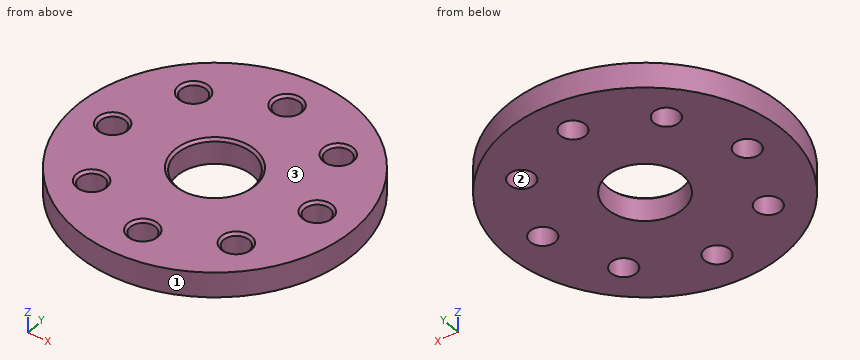
```python
from build123d import *

# Parameters (mm, degrees)
SKETCH1_R           = 11
BOSS_EXTRUDE1_DEPTH = 2
SKETCH3_R           = 3
CUT_EXTRUDE1_DEPTH  = 16.684387141
SKETCH4_R           = 1
CUT_EXTRUDE2_DEPTH  = 16.684387141
CHAMFER1_SIZE       = 0.2
CHAMFER2_SIZE       = 0.2
CIRPATTERN1_COUNT   = 8
CHAMFER4_SIZE       = 0.2
CHAMFER5_SIZE       = 0.2
CHAMFER6_SIZE       = 0.2


with BuildPart() as part:
    # Sketch1 → Boss-Extrude1 (new body)
    with BuildSketch(Plane.XY):
        Circle(SKETCH1_R)
    extrude(amount=BOSS_EXTRUDE1_DEPTH)

    # Sketch3 → Cut-Extrude1 (cut, through all)
    with BuildSketch(Plane.XY.offset(2)):
        Circle(SKETCH3_R)
    extrude(amount=-CUT_EXTRUDE1_DEPTH, mode=Mode.SUBTRACT)

    # Sketch4 → Cut-Extrude2 (cut, through all)
    with BuildSketch(Plane.XY.offset(2)):
        with Locations((0, 8)):
            Circle(SKETCH4_R)
    cut_extrude2 = extrude(amount=-CUT_EXTRUDE2_DEPTH, mode=Mode.SUBTRACT)

    # Chamfer1
    chamfer1_edges = [part.edges().sort_by_distance(p)[0] for p in [
        (-1, 8, 2),
    ]]
    chamfer(chamfer1_edges, length=CHAMFER1_SIZE)

    # Chamfer2
    chamfer2_edges = [part.edges().sort_by_distance(p)[0] for p in [
        (-3, 0, 2),
    ]]
    chamfer(chamfer2_edges, length=CHAMFER2_SIZE)

    # CirPattern1: Cut-Extrude2 ×8 about axis
    cirpattern1_axis = Axis((0, 0, 0), (0, 0, 1))
    for i in range(1, CIRPATTERN1_COUNT):
        add(cut_extrude2.rotate(cirpattern1_axis, i * 360 / CIRPATTERN1_COUNT), mode=Mode.SUBTRACT)

    # Chamfer4
    chamfer4_edges = [part.edges().sort_by_distance(p)[0] for p in [
        (-4.949747468, -6.363961031, 2),
    ]]
    chamfer(chamfer4_edges, length=CHAMFER4_SIZE)

    # Chamfer5
    chamfer5_edges = [part.edges().sort_by_distance(p)[0] for p in [
        (8, 1, 2),
        (4.949747468, 6.363961031, 2),
    ]]
    chamfer(chamfer5_edges, length=CHAMFER5_SIZE)

    # Chamfer6
    chamfer6_edges = [part.edges().sort_by_distance(p)[0] for p in [
        (-6.363961031, 4.949747468, 2),
        (-8, -1, 2),
        (1, -8, 2),
        (6.363961031, -4.949747468, 2),
    ]]
    chamfer(chamfer6_edges, length=CHAMFER6_SIZE)


solid = part.part
```
Verification items for the finished model (mm, model axes). Face numbers are marked on the shaded views. Round coordinates to 2 decimals unless told otherwise and drop trailing zeros. Order: outer loops, then holes, each group sorted by start corner. A loop starts at its lowest first (then second) coordinate and runs counter-clockwise, first axis right, second up. Notation, with made-up numbers: (42, -18.75) -> (94, -18.75) arc R21 cw to (94, 8.25) -> close; hole circle Ø3 at (-3, 30). An arc over 180 degrees is marked (long way). Put each result on its own line as item: value. Start each with the question number.
(1) Draft check along Y on the marked faces 1, 2 and 3. Enter one of: +Y half, -Y half, draft (parallel to the pull), parting line (faces both ways), or undercut.
(2) Section check A-A (y = 0). Enter the section's corners in (x, z), then the cut area to 3 significant figures.
(3) Section check C-C (z = 1.1). State how many separate pieces and enclosed holes the cut face has, then the cut area to 3 significant figures.
(4) Depth check by flat-ended pin: pin 1 Ø1.6 at (x, y) = (5.66, 5.66) entering from +Z. Enter the tip coordinate at first touch or a pass-through.
(5) Section check D-D (x = 8). Enter the section's corners in (y, z), then the cut area to 3 significant figures.
(6) Material ranges on line 1 along Y through (x, z) = (0, 1.4); line 2 along Y through (x, z) = (-6, 0.1); line 3 along Y through (x, z) = (6.25, 1.65), recorded low to high.
Completed:
1. face 1: parting line
1. face 2: undercut
1. face 3: draft
2. outline: (-11, 0) -> (-9, 0) -> (-9, 1.8) -> (-9.2, 2) -> (-11, 2) -> close; (-7, 0) -> (-3, 0) -> (-3, 1.8) -> (-3.2, 2) -> (-6.8, 2) -> (-7, 1.8) -> close; (3, 0) -> (7, 0) -> (7, 1.8) -> (6.8, 2) -> (3.2, 2) -> (3, 1.8) -> close; (9, 0) -> (11, 0) -> (11, 2) -> (9.2, 2) -> (9, 1.8) -> close
2. area: 23.9 mm2
3. separate pieces: 1
3. enclosed holes: 9
3. area: 327 mm2
4. pin 1: passes through
5. outline: (-7.55, 0) -> (-1, 0) -> (-1, 1.8) -> (-1.2, 2) -> (-7.55, 2) -> close; (1, 0) -> (7.55, 0) -> (7.55, 2) -> (1.2, 2) -> (1, 1.8) -> close
5. area: 26.2 mm2
6. line 1: y = -11 to -9, -7 to -3, 3 to 7, 9 to 11
6. line 2: y = -9.22 to -6.6, -4.72 to 4.72, 6.6 to 9.22
6. line 3: y = -9.05 to -6.46, -4.85 to 4.85, 6.46 to 9.05
